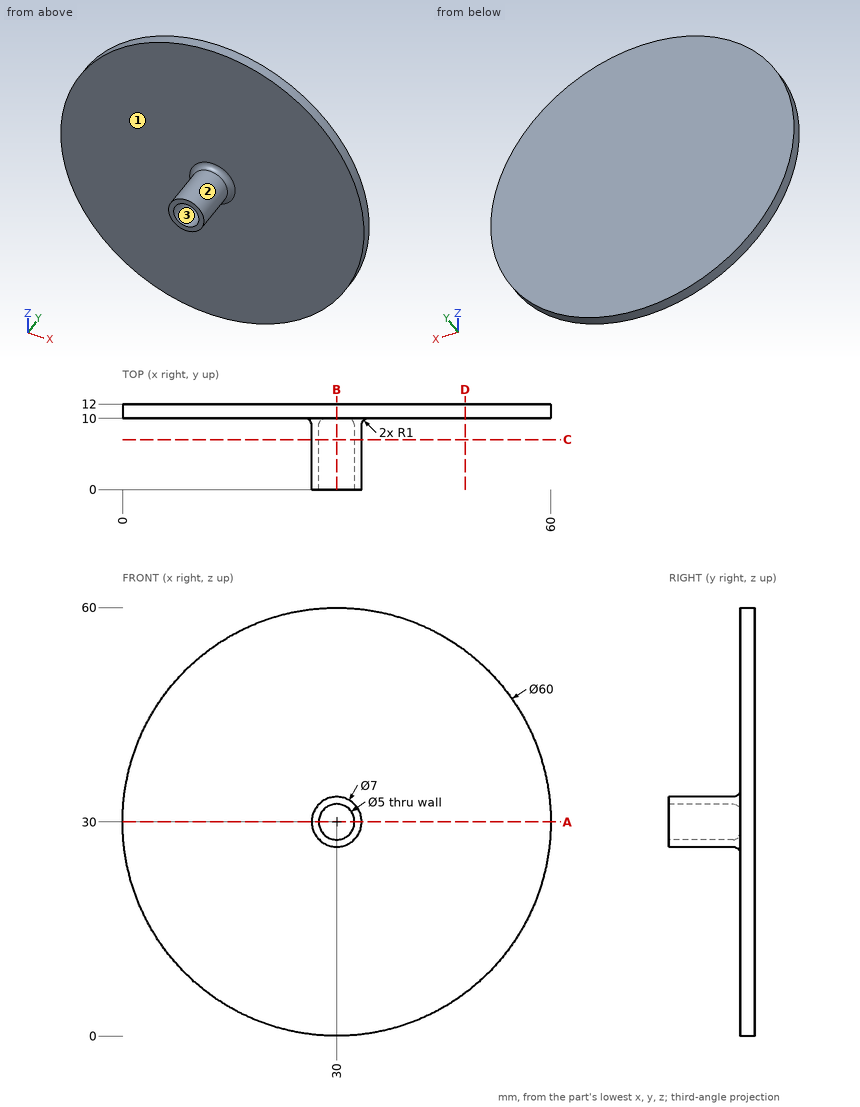
Here's the drawing with two shaded views (mm, measured from the low corner). I have some questions. Give positions to 0.01 mm unless a question says otherwise; leave off trailing zeros. Order: outer loops, then holes, each group sorted by start corner. A loop starts at its lowest first (then second) coordinate and runs counter-clockwise, first axis right, second up. Notation, with made-up numbers: M 54.25,77 L 78.25,77 A31 ccw 78.25,102 Z; hole C -11.5,1 d4. An arc over 180 degrees is marked long. One line per item, written item: value.
1) I want a section at A-A, the plane z = 30. List the corners of the cut face in (x, y) for me.
Answer sheet:
outline: M 0,10 L 25.5,10 A1 cw 26.5,9 L 26.5,0 L 27.5,0 L 27.5,9 A1 cw 28.5,10 L 31.5,10 A1 cw 32.5,9 L 32.5,0 L 33.5,0 L 33.5,9 A1 cw 34.5,10 L 60,10 L 60,12 L 0,12 Z
2) I want a section at B-B, the plane x = 30. List the corners of the cut face in (y, z) for me.
Answer sheet:
outline: M 0,26.5 L 9,26.5 A1 cw 10,25.5 L 10,0 L 12,0 L 12,60 L 10,60 L 10,34.5 A1 cw 9,33.5 L 0,33.5 L 0,32.5 L 9,32.5 A1 cw 10,31.5 L 10,28.5 A1 cw 9,27.5 L 0,27.5 Z
3) We'd pull the mould along Z, two halves only. Please class the marked faces 1, 2 and 3: released by +Z, released by -Z, zero draft, split by the parting line, or undercut.
Answer sheet:
face 1: zero draft
face 2: split by the parting line
face 3: undercut
4) For P1, Ø3.5, axis at x = 30, z = 29.5, coming from the -Y side; P2, Ø3, axis at x = 30, z = 30, coming from the -Y side; P3, Ø6, axis at y = 8.5, z = 15.5, coming from the +X side, each with a flat end and sliding along its axis, tell me the tip position at first contact or that it passes through.
Answer sheet:
P1: stops at y = 9.66
P2: stops at y = 10
P3: stops at x = 57.54
5) Please list where these lines run through material, in increasing order: line 1 along X through (y, z) = (6.75, 30); line 2 along Y through (x, z) = (36, 7); line 3 along X through (y, z) = (10.5, 24).
Answer sheet:
line 1: x = 26.5 to 27.5, 32.5 to 33.5
line 2: y = 10 to 12
line 3: x = 0.61 to 59.39
6) I want a section at C-C, the plane y = 7. List the corners of the cut face in (x, z) for me.
Answer sheet:
outline: C 30,30 d7; hole C 30,30 d5
7) I want a section at D-D, the plane x = 48. List the corners of the cut face in (y, z) for me.
Answer sheet:
outline: M 10,6 L 12,6 L 12,54 L 10,54 Z
